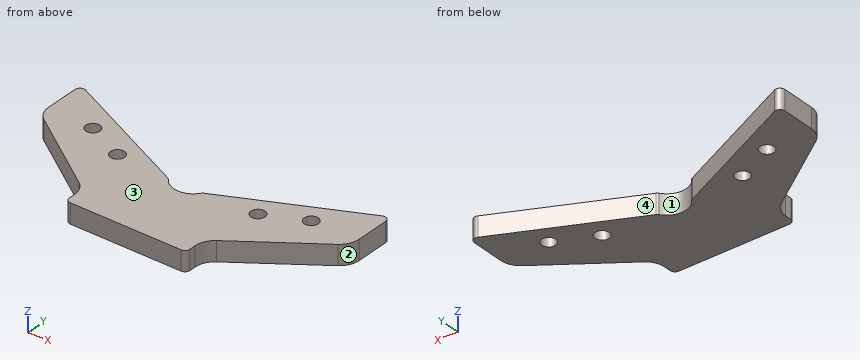
from build123d import *

# Parameters (mm, degrees)
EXTRUDE1_DEPTH         = 12
M10_GEVINDHULLER_D     = 8.5
M10_GEVINDHULLER_DEPTH = 22
M10_GEVINDHULLER_TIP   = 2.553657631


with BuildPart() as part:
    # Sketch1 → Extrude1 (new body)
    with BuildSketch(Plane.XY):
        with BuildLine():
            Line((36.5, 6.991261946), (36.5, 3))
            ThreePointArc((36.5, 3), (35.621320344, 0.878679656), (33.5, 0))
            Line((33.5, 0), (0, 0))
            Line((0, 0), (-33.5, 0))
            ThreePointArc((-33.5, 0), (-35.621320344, 0.878679656), (-36.5, 3))
            Line((-36.5, 3), (-36.5, 6.991261946))
            ThreePointArc((-36.5, 6.991261946), (-37.855870002, 12.532245305), (-41.617082764, 16.821086478))
            Line((-41.617082764, 16.821086478), (-88.882917236, 49.916980075))
            ThreePointArc((-88.882917236, 49.916980075), (-92.644129998, 54.205821248), (-94, 59.746804607))
            Line((-94, 59.746804607), (-94, 80))
            ThreePointArc((-94, 80), (-92.611898825, 82.530174337), (-89.732145215, 82.718923361))
            Line((-89.732145215, 82.718923361), (-11.04340479, 46.02576109))
            ThreePointArc((-11.04340479, 46.02576109), (-10.379689702, 45.602276211), (-9.84900766, 45.020697556))
            ThreePointArc((-9.84900766, 45.020697556), (0, 39.876136865), (9.84900766, 45.020697556))
            ThreePointArc((9.84900766, 45.020697556), (10.379689702, 45.602276211), (11.04340479, 46.02576109))
            Line((11.04340479, 46.02576109), (89.732145215, 82.718923361))
            ThreePointArc((89.732145215, 82.718923361), (92.611898825, 82.530174337), (94, 80))
            Line((94, 80), (94, 59.746804607))
            ThreePointArc((94, 59.746804607), (92.644129998, 54.205821248), (88.882917236, 49.916980075))
            Line((88.882917236, 49.916980075), (41.617082764, 16.821086478))
            ThreePointArc((41.617082764, 16.821086478), (37.855870002, 12.532245305), (36.5, 6.991261946))
        make_face()
    extrude(amount=EXTRUDE1_DEPTH)

    # M10 gevindhuller
    with Locations(Plane.XY.offset(12)):
        with Locations((-66.064002463, 58.441752114), (-42.5, 47.453677309), (66.064002463, 58.441752114), (42.5, 47.453677309)):
            Hole(M10_GEVINDHULLER_D / 2, depth=M10_GEVINDHULLER_DEPTH)
            with Locations((0, 0, -(M10_GEVINDHULLER_DEPTH + M10_GEVINDHULLER_TIP / 2))):  # 118° drill point
                Cone(0, M10_GEVINDHULLER_D / 2, M10_GEVINDHULLER_TIP, mode=Mode.SUBTRACT)


solid = part.part
Design review of the part built by this model. Coordinates are the model's own, in mm. Face numbers are marked on the shaded views. Give positions to 0.01 mm unless a question says otherwise; leave off trailing zeros. Loops run counter-clockwise (first coordinate to the right, second up) from the corner with the lowest first, then second, coordinate; pieces in that order, holes last. Notation, with made-up numbers: (-26, 47) - (7, 47) arc R6 ccw to (7, 55) - close; hole circle Ø9 at (20.25, 26). An arc over 180 degrees is marked (long way). Write item = value, one per line.
1) Clearance check with flat-ended pins moving along their axes: pin 1 Ø1.2 at (y, z) = (5.5, 8.5) entering from -X; pin 2 Ø11 at (x, y) = (-66.06, 58.44) entering from -Z; pin 3 Ø2 at (x, z) = (17, 9) entering from +Y; pin 4 Ø3 at (y, z) = (18, 4) entering from -X. State where each tip first meets the part, or that it passes through.
Result sheet:
pin_1 = -36.5
pin_2 = 0
pin_3 = 49.27
pin_4 = -45.44
2) Take a section at B-B on x = 77.5. State the section outline as (y, z) points.
Result sheet:
outline = (41.95, 0) - (77.01, 0) - (77.01, 12) - (41.95, 12) - close
3) To check wall thickness, follow line 1 (Y direction, x = -68.5, z = 10.25); line 2 (X direction, y = 73, z = 1); line 3 (X direction, y = 3, z = 10). State the ranges of each line that lie inside material, in increasing order.
Result sheet:
line_1 = 35.64 to 54.96, 61.92 to 72.82
line_2 = -94 to -68.89, 68.89 to 94
line_3 = -36.5 to 36.5
4) Draft analysis for pull direction X (two halves, no side actions). For the marked faces 1, 2, 3 and 4, state which applies: +X half, -X half, draft (parallel to the pull), parting line (faces both ways), or undercut.
Result sheet:
face_1 = undercut
face_2 = +X half
face_3 = draft
face_4 = undercut
5) Take a section at A-A on z = 1.75. State the section outline as (x, y) points.
Result sheet:
outline = (-94, 59.75) arc R12 ccw to (-88.88, 49.92) - (-41.62, 16.82) arc R12 cw to (-36.5, 6.99) - (-36.5, 3) arc R3 ccw to (-33.5, 0) - (33.5, 0) arc R3 ccw to (36.5, 3) - (36.5, 6.99) arc R12 cw to (41.62, 16.82) - (88.88, 49.92) arc R12 ccw to (94, 59.75) - (94, 80) arc R3 ccw to (89.73, 82.72) - (11.04, 46.03) arc R3 ccw to (9.85, 45.02) arc R12 cw to (-9.85, 45.02) arc R3 ccw to (-11.04, 46.03) - (-89.73, 82.72) arc R3 ccw to (-94, 80) - close; hole circle Ø8.5 at (-66.06, 58.44); hole circle Ø8.5 at (-42.5, 47.45); hole circle Ø8.5 at (42.5, 47.45); hole circle Ø8.5 at (66.06, 58.44)
6) Take a section at C-C on x = -82.5. State the section outline as (y, z) points, and give its area (3 significant figures).
Result sheet:
outline = (45.45, 0) - (79.35, 0) - (79.35, 12) - (45.45, 12) - close
area = 407 mm2
